Build history of the part. All positions in model axes, mm. A direction names the side the tool comes from. Give positions to 0.01 mm unless a question says otherwise; leave off trailing zeros. Order: outer loops, then holes, each group sorted by start corner. A loop starts at its lowest first (then second) coordinate and runs counter-clockwise, first axis right, second up. Notation, with made-up numbers: M 49.25,63.25 L 68.25,63.25 A28 cw 68.25,91.25 Z; hole C 87,67.25 d5. An arc over 180 degrees is marked long. Use CSV: the item, a comma, the result in double quotes. Start each with the question number.
Item 1: Pin check, flat tips, straight feed: P1, Ø3, axis at y = 19, z = 1, coming from the +X side; P2, Ø10, axis at x = 15, y = 40, coming from the -Z side; P3, Ø4, axis at x = 1, y = 32, coming from the -Z side; P4, Ø23, axis at x = -14.5, z = 14.5, coming from the -Y side. Stop position of each tip, or through.
Item 2: Band-saw the part on A-A on x = 0. Write the cut outline in (y, z).
Item 3: Band-saw the part on D-D on z = -28. Write the cut outline in (x, y).
Item 4: Band-saw the part on C-C on y = 65.5. Write the cut outline in (x, z), plus the area to 3 significant figures.
Item 5: Two-plate mould, pull along Y, no slides. Class faces 4 (the flat face through (11.34, 47, 27.41)), 5 (the flat face through (18, 77, -18)), 6 (the cylindrical face through (-30.736, 52.577, 4.036)): pulls with the +Y half, pulls with the -Y half, needs draft (parallel to the pull), parting line crosses it, or undercut.
Item 6: Band-saw the part on B-B on z = 0. Write the cut outline in (x, y).
Item 7: Which spindle directions (+Z, -Z, +X, -X, +Y, -Y) get a long thin tool onto all of the face, cutting with end or side? Do faces 1 (the flat face through (27.41, 10, -11.34)), 2 (the cylindrical face through (-30.736, 5.07, 4.036)), 3 (the flat face through (-21.1, 0, -7.3)). Say none if no direction does.
Item 8: Wall check: line 1 along X through (y, z) = (54.5, 0); line 2 along Y through (x, z) = (20.5, 22.5); line 3 along X through (y, z) = (34, 0). Give the ranges that are in metal, low to high.
from build123d import *


with BuildPart() as part:
    # Sketch1 → Revolve1 (revolve)
    with BuildSketch(Plane.XY, mode=Mode.PRIVATE) as revolve1_sk:
        Polygon((22, 0), (31, 0), (31, 10), (29.5, 10), (29.5, 47), (31, 47), (31, 58), (38, 58), (38, 69), (41.5, 69), (41.5, 77), (22, 77), align=None)
    revolve(revolve1_sk.sketch.rotate(Axis((0, 0, 0), (0, 1, 0)), 90), axis=Axis((0, 0, 0), (0, 1, 0)))  # turned: the seam where the file's is


solid = part.part
Model answer:
1,P1,"stops at x = 29.5"
1,P2,"stops at z = -27.75"
1,P3,"stops at z = -29.5"
1,P4,"stops at y = 0"
2,outline,"M 0,-31 L 10,-31 L 10,-29.5 L 47,-29.5 L 47,-31 L 58,-31 L 58,-38 L 69,-38 L 69,-41.5 L 77,-41.5 L 77,-22 L 0,-22 Z; M 0,22 L 77,22 L 77,41.5 L 69,41.5 L 69,38 L 58,38 L 58,31 L 47,31 L 47,29.5 L 10,29.5 L 10,31 L 0,31 Z"
3,outline,"M -30.63,69 L -25.69,69 L -25.69,58 L -13.3,58 L -13.3,47 L -9.29,47 L -9.29,10 L -13.3,10 L -13.3,0 L 13.3,0 L 13.3,10 L 9.29,10 L 9.29,47 L 13.3,47 L 13.3,58 L 25.69,58 L 25.69,69 L 30.63,69 L 30.63,77 L -30.63,77 Z"
4,outline,"C 0,0 d76; hole C 0,0 d44"
4,area,"3,020 mm^2"
5,face 4,"undercut"
5,face 5,"pulls with the +Y half"
5,face 6,"needs draft"
6,outline,"M -41.5,69 L -38,69 L -38,58 L -31,58 L -31,47 L -29.5,47 L -29.5,10 L -31,10 L -31,0 L -22,0 L -22,77 L -41.5,77 Z; M 22,0 L 31,0 L 31,10 L 29.5,10 L 29.5,47 L 31,47 L 31,58 L 38,58 L 38,69 L 41.5,69 L 41.5,77 L 22,77 Z"
7,face 1,"none"
7,face 2,"-Y"
7,face 3,"+Z, -Z, +X, -X, -Y"
8,line 1,"x = -31 to -22, 22 to 31"
8,line 2,"y = 0 to 10, 47 to 77"
8,line 3,"x = -29.5 to -22, 22 to 29.5"
